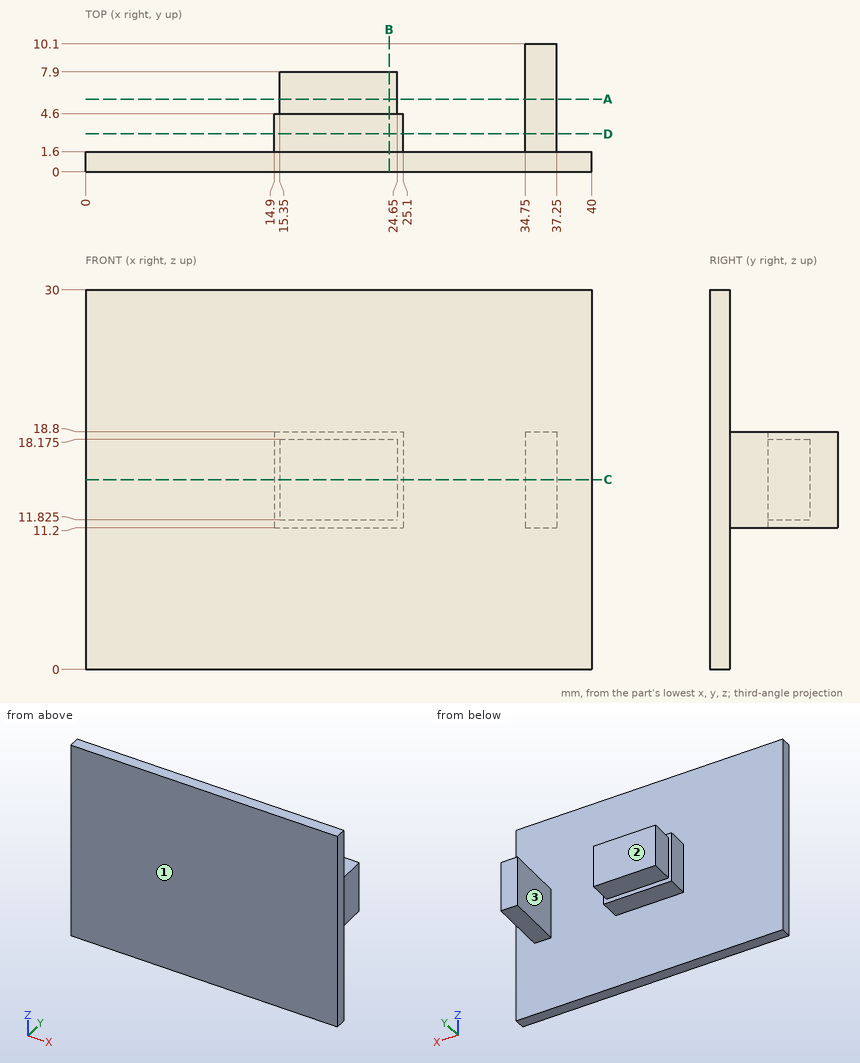
Design review of the part shown in the three views and the two pictorial views. Dimensions are in mm from the part's minimum x, y and z. A direction names the side the tool comes from. Coordinates: 2 decimals unless noted, no trailing zeros. Loops run counter-clockwise (first coordinate to the right, second up) from the corner with the lowest first, then second, coordinate; pieces in that order, holes last. Notation, with made-up numbers: M 7.25,89.5 L 53.25,89.5 A21 ccw 53.25,124.5 Z; hole C 72,47.25 d4. An arc over 180 degrees is marked long. Put each result on its own line as item: value. Start each with the question number.
Q1. Add section D-D (y = 3). Write out the cut boundary in (x, z).
Q2. Add section B-B (x = 24). Write out the cut boundary in (y, z) (3 decimals).
Q3. Clearance check with flat-ended pins moving along their axes: pin 1 (1.6 mm diameter, centred on y = 6, z = 16.5, fed in from -X); pin 2 (3.5 mm diameter, centred on x = 22, y = 6, fed in from -Z); pin 3 (3.5 mm diameter, centred on y = 6, z = 15.5, fed in from +X); pin 4 (4 mm diameter, centred on x = 27.5, y = 7, fed in from -Z). State where each tip first meets the part, or that it passes through.
Q4. Wall thickness on line 1 (X direction, y = 2.5, z = 18); line 2 (X direction, y = 5.5, z = 16); line 3 (Y direction, x = 16, z = 7): over which ranges is each line inside the solid? List them lowest first.
Q5. For the marked faces 1, 2 and 3, list the 3-axis set-ups (+Z, -Z, +X, -X, +Y, -Y) from which the entire face can be reached by the end or side of a thin tool; tool diameter is ignored.
Q6. Add section C-C (z = 15). Write out the cut boundary in (x, y), and give its area (3 significant figures).
Q7. Add section A-A (y = 5.75). Write out the cut boundary in (x, z) (3 decimals), and give its area (3 significant figures).
Answers:
1. outline: M 14.9,11.2 L 25.1,11.2 L 25.1,18.8 L 14.9,18.8 Z; M 34.75,11.2 L 37.25,11.2 L 37.25,18.8 L 34.75,18.8 Z
2. outline: M 0,0 L 1.6,0 L 1.6,11.2 L 4.6,11.2 L 4.6,11.825 L 7.9,11.825 L 7.9,18.175 L 4.6,18.175 L 4.6,18.8 L 1.6,18.8 L 1.6,30 L 0,30 Z
3. pin 1: stops at x = 15.35
3. pin 2: stops at z = 11.2
3. pin 3: stops at x = 37.25
3. pin 4: passes through
4. line 1: x = 14.9 to 25.1, 34.75 to 37.25
4. line 2: x = 15.35 to 24.65, 34.75 to 37.25
4. line 3: y = 0 to 1.6
5. face 1: +Z, -Z, +X, -X, -Y
5. face 2: +Z, -Z, -X, +Y
5. face 3: +Z, -Z, +Y
6. outline: M 0,0 L 40,0 L 40,1.6 L 37.25,1.6 L 37.25,10.1 L 34.75,10.1 L 34.75,1.6 L 25.1,1.6 L 25.1,4.6 L 24.65,4.6 L 24.65,7.9 L 15.35,7.9 L 15.35,4.6 L 14.9,4.6 L 14.9,1.6 L 0,1.6 Z
6. area: 147 mm^2
7. outline: M 15.35,11.825 L 24.65,11.825 L 24.65,18.175 L 15.35,18.175 Z; M 34.75,11.2 L 37.25,11.2 L 37.25,18.8 L 34.75,18.8 Z
7. area: 78.1 mm^2
